```python
from build123d import *

# Parameters (mm, degrees)
F0_R     = 0.6
F1_DEPTH = 3
F2_W     = 3.05
F2_H     = 6
F3_DEPTH = 3
F5_D     = 1
F6_R     = 1


with BuildPart() as f1:
    # F0 (on Top) → F1 (new body)
    with BuildSketch(Plane.XY):
        Polygon((-20, 13.2), (-20, -13.2), (0, -13.2), (20, -13.2), (20, 13.2), align=None)
        with Locations((-13.875, 0)):
            Circle(F0_R, mode=Mode.SUBTRACT)
        Polygon((-14.05, 6.15), (-14.05, 9.25), (14.05, 9.25), (14.05, 6.15), (11.5, 6.15), (11.5, -6.15), (14.05, -6.15), (14.05, -9.25), (-14.05, -9.25), (-14.05, -6.15), (-11.5, -6.15), (-11.5, 6.15), align=None, mode=Mode.SUBTRACT)
        with Locations((13.875, 0)):
            Circle(F0_R, mode=Mode.SUBTRACT)
    extrude(amount=F1_DEPTH)

    # F2 (on face) → F3 (join, through all)
    with BuildSketch(Plane(origin=(0, 0, 0), x_dir=(1, 0, 0), z_dir=(0, 0, -1))):
        with Locations((-21.525, 0)):
            Rectangle(F2_W, F2_H)
        with Locations((21.525, 0)):
            Rectangle(F2_W, F2_H)
    extrude(amount=-F3_DEPTH)

    # F5 (through all)
    with Locations(Plane.XY.offset(3)):
        with Locations((-14.05, 9.25), (-14.05, 6.15), (-20, 3), (-20, -3), (-14.05, -6.15), (-14.05, -9.25), (14.05, -6.15), (14.05, -9.25), (20, -3), (20, 3), (14.05, 6.15), (14.05, 9.25)):
            Hole(F5_D / 2)

    # F6
    f6_edges = [f1.edges().sort_by_distance(p)[0] for p in [
        (-20, 13.2, 1.5),
        (-23.05, 3, 1.5),
        (-23.05, -3, 1.5),
        (-20, -13.2, 1.5),
        (-11.5, 6.15, 1.5),
        (11.5, -6.15, 1.5),
        (11.5, 6.15, 1.5),
        (23.05, 3, 1.5),
        (20, 13.2, 1.5),
        (23.05, -3, 1.5),
        (20, -13.2, 1.5),
        (-11.5, -6.15, 1.5),
        (-20, 3.5, 1.5),
        (20, 3.5, 1.5),
        (20.5, 3, 1.5),
        (20.5, -3, 1.5),
        (20, -3.5, 1.5),
        (-20, -3.5, 1.5),
        (-20.5, -3, 1.5),
        (-20.5, 3, 1.5),
        (-13.55, 6.15, 1.5),
        (-13.55, -6.15, 1.5),
        (-14.05, -6.65, 1.5),
        (-14.05, -8.75, 1.5),
        (-13.55, -9.25, 1.5),
        (13.55, -9.25, 1.5),
        (14.05, -8.75, 1.5),
        (14.05, -6.65, 1.5),
        (13.55, -6.15, 1.5),
        (13.55, 6.15, 1.5),
        (14.05, 6.65, 1.5),
        (14.05, 8.75, 1.5),
        (13.55, 9.25, 1.5),
        (-13.55, 9.25, 1.5),
        (-14.05, 8.75, 1.5),
        (-14.05, 6.65, 1.5),
    ]]
    fillet(f6_edges, radius=F6_R)


solid = f1.part
```
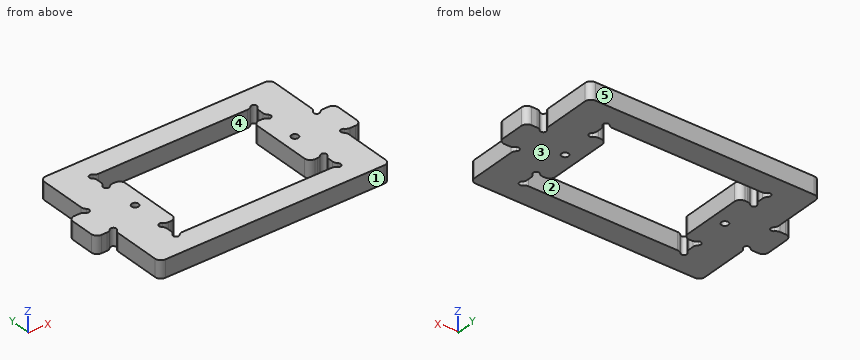
Check sheet for the modelled part. Datum: model origin and axes. Units: mm. Face numbers are marked on the shaded views. A direction names the side the tool comes from. Give positions to 0.01 mm unless a question says otherwise; leave off trailing zeros. Order: outer loops, then holes, each group sorted by start corner. A loop starts at its lowest first (then second) coordinate and runs counter-clockwise, first axis right, second up. Notation, with made-up numbers: (51, 47.25) -> (83, 47.25) arc R31 ccw to (83, 75.25) -> close; hole circle Ø7 at (36, 49). An arc over 180 degrees is marked (long way). Use CSV: the item, a comma, the result in double quotes. Start each with the question number.
1) Sectioned sample at A-A, the plane y = 0. Record the boundary of the cut face in (x, z) (3 decimals).
2) Mould release check, pull along Y, two halves, no side actions. Record for the marked faces 1, 2 and 3: released by +Y, released by -Y, zero draft, split by the parting line, or undercut.
3) Go/stop test with flat-tipped pins: P1, Ø10, axis at x = 4, y = -4, coming from the +Z side; P2, Ø0.5, axis at x = -21.5, z = 1.5, coming from the -Y side; P3, Ø0.7, axis at x = 21.5, z = 2, coming from the +Y side; P4, Ø0.7, axis at y = -8, z = 1, coming from the -X side. Record where each tip stops, or that it passes through.
4) Sectioned sample at C-C, the plane z = 0.55. Give the number of separate pieces and of enclosed holes in the cut face, plus the area to 3 significant figures.
5) Sectioned sample at B-B, the plane x = -12. Record the boundary of the cut face in (y, z), plus the area to 3 significant figures.
6) Set-up check for the marked faces 4 and 5: record each of +Z, -Z, +X, -X, +Y, -Y from which the full face is reachable in a straight line by a thin tool's end or side.
7) Material ranges on line 1 (Y direction, x = 3.5, z = 1.05); line 2 (X direction, y = 0.5, z = 1.35); line 3 (X direction, y = 6, z = 0.9), recorded low to high. Write a range as from..to.
Recorded:
1,outline,"(-23.05, 0) -> (-14.475, 0) -> (-14.475, 3) -> (-23.05, 3) -> close; (-13.275, 0) -> (-11.5, 0) -> (-11.5, 3) -> (-13.275, 3) -> close; (11.5, 0) -> (13.275, 0) -> (13.275, 3) -> (11.5, 3) -> close; (14.475, 0) -> (23.05, 0) -> (23.05, 3) -> (14.475, 3) -> close"
2,face 1,"released by -Y"
2,face 2,"undercut"
2,face 3,"zero draft"
3,P1,"through"
3,P2,"y = -3"
3,P3,"y = 3"
3,P4,"x = -20"
4,separate pieces,"1"
4,enclosed holes,"3"
4,area,"622 mm2"
5,outline,"(-13.2, 0) -> (-9.25, 0) -> (-9.25, 3) -> (-13.2, 3) -> close; (-6.02, 0) -> (6.02, 0) -> (6.02, 3) -> (-6.02, 3) -> close; (9.25, 0) -> (13.2, 0) -> (13.2, 3) -> (9.25, 3) -> close"
5,area,"59.8 mm2"
6,face 4,"+Z, -Z"
6,face 5,"+Z, -Z, +X, -X, +Y"
7,line 1,"-13.2..-9.25, 9.25..13.2"
7,line 2,"-23.05..-14.21, -13.54..-11.5, 11.5..13.54, 14.21..23.05"
7,line 3,"-20..-14.53, -13.46..-11.97, 11.97..13.46, 14.53..20"
